Study the drawing (mm; zero at the part's minimum x, y, z) and answer. Give positions to 0.01 mm unless a question says otherwise; leave off trailing zeros. Order: outer loops, then holes, each group sorted by start corner. A loop starts at its lowest first (then second) coordinate and runs counter-clockwise, first axis right, second up. Notation, with made-up numbers: (-17.75, 84.5) - (36.25, 84.5) arc R20 ccw to (36.25, 110.5) - close; hole circle Ø11 at (74.25, -1.75). An arc over 180 degrees is marked (long way). Put each result on its own line as item: value.
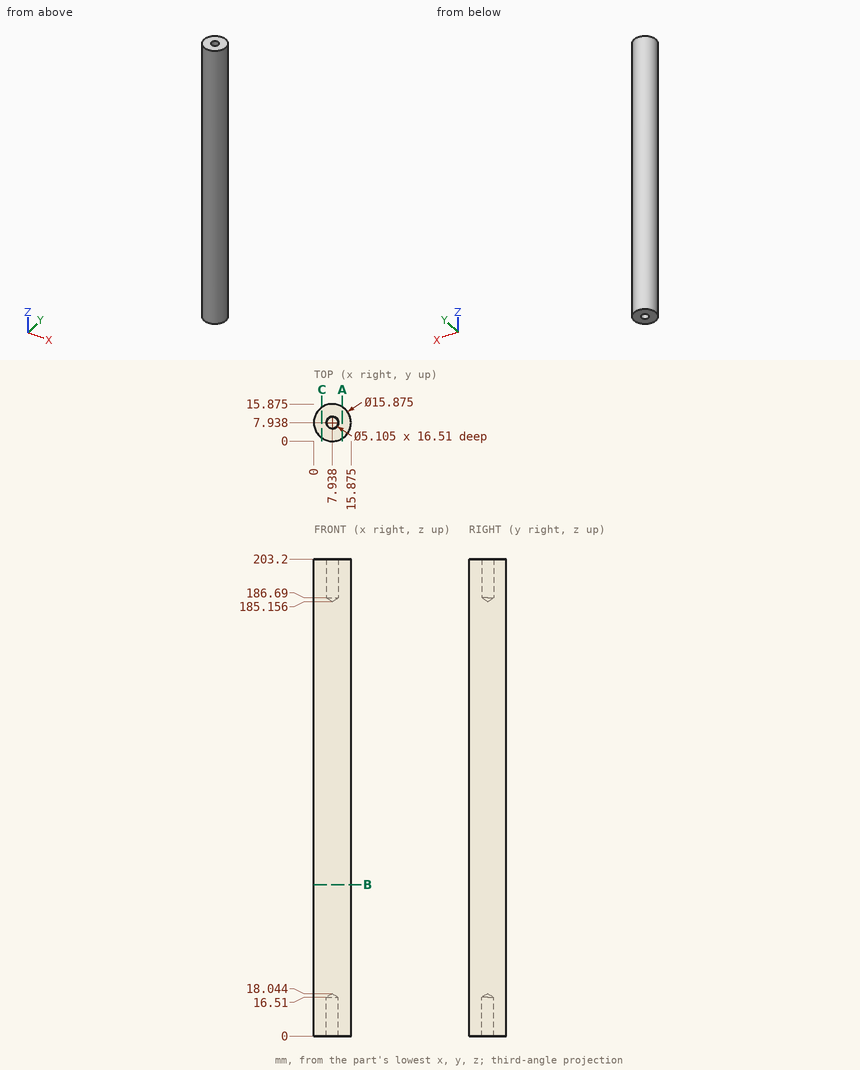
(1) Straight lines are drawn through the part: line 1 (Y direction, x = 7.5, z = 177); line 2 (X direction, y = 8.25, z = 93); line 3 (Z direction, x = 7.5, y = 7.5). For each, find the intervals that lie inside material, in ascending order.
Geometry check:
line 1: y = 0.01 to 15.86
line 2: x = 0.01 to 15.87
line 3: z = 17.67 to 185.53
(2) Section B-B, the plane z = 64.5 is taken. Write down the section's boundary in (x, y) (1 decimal).
Geometry check:
outline: circle Ø15.9 at (7.9, 7.9)
(3) Section C-C, the plane x = 3.5 is taken. Write down the section's boundary in (y, z).
Geometry check:
outline: (1.36, 0) - (14.52, 0) - (14.52, 203.2) - (1.36, 203.2) - close
(4) Section A-A, the plane x = 12.25 is taken. Write down the section's boundary in (y, z).
Geometry check:
outline: (1.27, 0) - (14.6, 0) - (14.6, 203.2) - (1.27, 203.2) - close
(5) Given pin 1 (1.5 mm diameter, centred on y = 2.5, z = 90.5, fed in from -X); pin 2 (1 mm diameter, centred on y = 7.5, z = 71, fed in from +X) (1 decimal); pin 3 (5 mm diameter, centred on x = 4, z = 177.5, fed in from +Y); pin 4 (2 mm diameter, centred on x = 10.5, z = 151.5, fed in from -Y) (1 decimal), each flat-ended and moving along its own axis, determine where each tip first touches the part or whether it passes through.
Geometry check:
pin 1: stops at x = 1.53
pin 2: stops at x = 15.9
pin 3: stops at y = 15.74
pin 4: stops at y = 0.2
